from build123d import *

# Parameters (mm, degrees)
SKETCH_1_R          = 1.35
EXTRUDE_1_DEPTH     = 10
SKETCH_2_W          = 110
SKETCH_2_H          = 30
EXTRUDE_2_DEPTH     = 26
CUT_EXTRUDE_1_DEPTH = 76.432088663
EXTRUDE_3_DEPTH     = 7
SKETCH_5_R          = 1.35
CUT_EXTRUDE_2_DEPTH = 7
SKETCH_6_W          = 65
SKETCH_6_H          = 6
EXTRUDE_4_DEPTH     = 4
SKETCH_7_W          = 3.3
SKETCH_7_H          = 30
SKETCH_7_W_2        = 2.7
EXTRUDE_5_DEPTH     = 9
RIB_1_REACH         = 79.332
SKETCH_8_WALL_W     = 169.39207434
SKETCH_8_WALL_H     = 10
RIB_2_REACH         = 79.332
SKETCH_9_WALL_W     = 167.056457124
SKETCH_9_WALL_H     = 10
CUT_EXTRUDE_3_REACH = 124.7
SKETCH_10_R         = 1.75
CUT_EXTRUDE_4_REACH = 124.7
SKETCH_11_R         = 1.75
FILLET_1_R          = 2
CUT_EXTRUDE_5_DEPTH = 22
CHAMFER_1_SIZE      = 5
CHAMFER_2_SIZE      = 2
SKETCH_13_R         = 1.75
CUT_EXTRUDE_6_DEPTH = 72.973953622
CHAMFER_3_SIZE      = 5
SKETCH_14_R         = 3
CUT_EXTRUDE_7_DEPTH = 4


with BuildPart() as part:
    # 草图1 → 凸台-拉伸1 (new body)
    with BuildSketch(Plane(origin=(0, 0, 0), x_dir=(1, 0, 0), z_dir=(0, 1, 0))):
        with BuildLine():
            Line((10, 15), (55, 15))
            Line((55, 15), (55, -15))
            Line((55, -15), (10, -15))
            ThreePointArc((10, -15), (6.464466094, -16.464466094), (5, -20))
            Line((5, -20), (5, -25.5))
            ThreePointArc((5, -25.5), (3.535533906, -29.035533906), (0, -30.5))
            Line((0, -30.5), (-30, -30.5))
            ThreePointArc((-30, -30.5), (-33.535533906, -29.035533906), (-35, -25.5))
            Line((-35, -25.5), (-35, -20))
            ThreePointArc((-35, -20), (-36.464466094, -16.464466094), (-40, -15))
            Line((-40, -15), (-55, -15))
            Line((-55, -15), (-55, 15))
            Line((-55, 15), (-40, 15))
            ThreePointArc((-40, 15), (-36.464466094, 16.464466094), (-35, 20))
            Line((-35, 20), (-35, 22))
            Line((-35, 22), (5, 22))
            Line((5, 22), (5, 20))
            ThreePointArc((5, 20), (6.464466094, 16.464466094), (10, 15))
        make_face()
        with Locations(Location((-30, 14.5, 0), (0, 0, 270))):
            Circle(SKETCH_1_R, mode=Mode.SUBTRACT)
        with Locations(Location((0, 14.5, 0), (0, 0, 270))):
            Circle(SKETCH_1_R, mode=Mode.SUBTRACT)
        with Locations(Location((0, -25.5, 0), (0, 0, 270))):
            Circle(SKETCH_1_R, mode=Mode.SUBTRACT)
        with Locations(Location((-30, -25.5, 0), (0, 0, 270))):
            Circle(SKETCH_1_R, mode=Mode.SUBTRACT)
    extrude(amount=EXTRUDE_1_DEPTH)

    # 草图2 → 凸台-拉伸2 (add)
    with BuildSketch(Plane(origin=(0, 10, 0), x_dir=(1, 0, 0), z_dir=(0, 1, 0))):
        Rectangle(SKETCH_2_W, SKETCH_2_H)
    extrude(amount=EXTRUDE_2_DEPTH)

    # 草图3 → 切除-拉伸1 (cut, through all)
    with BuildSketch(Plane.XY.offset(15)):
        with BuildLine():
            Line((-42, 30), (-28, 30))
            ThreePointArc((-28, 30), (-25.878679656, 29.121320344), (-25, 27))
            Line((-25, 27), (-25, 13))
            ThreePointArc((-25, 13), (-25.878679656, 10.878679656), (-28, 10))
            Line((-28, 10), (-42, 10))
            ThreePointArc((-42, 10), (-44.121320344, 10.878679656), (-45, 13))
            Line((-45, 13), (-45, 27))
            ThreePointArc((-45, 27), (-44.121320344, 29.121320344), (-42, 30))
        make_face()
        with BuildLine():
            Line((22, 10), (46, 10))
            ThreePointArc((46, 10), (48.121320344, 10.878679656), (49, 13))
            Line((49, 13), (49, 27))
            ThreePointArc((49, 27), (48.121320344, 29.121320344), (46, 30))
            Line((46, 30), (22, 30))
            ThreePointArc((22, 30), (19.878679656, 29.121320344), (19, 27))
            Line((19, 27), (19, 13))
            ThreePointArc((19, 13), (19.878679656, 10.878679656), (22, 10))
        make_face()
    extrude(amount=-CUT_EXTRUDE_1_DEPTH, mode=Mode.SUBTRACT)

    # 草图4 → 凸台-拉伸3 (add)
    with BuildSketch(Plane(origin=(0, 36, 0), x_dir=(1, 0, 0), z_dir=(0, 1, 0))):
        with BuildLine():
            Line((-28.5, 9), (39.5, 9))
            ThreePointArc((39.5, 9), (41.267766953, 8.267766953), (42, 6.5))
            Line((42, 6.5), (42, -6.5))
            ThreePointArc((42, -6.5), (41.267766953, -8.267766953), (39.5, -9))
            Line((39.5, -9), (-28.5, -9))
            ThreePointArc((-28.5, -9), (-30.267766953, -8.267766953), (-31, -6.5))
            Line((-31, -6.5), (-31, 6.5))
            ThreePointArc((-31, 6.5), (-30.267766953, 8.267766953), (-28.5, 9))
        make_face()
    extrude(amount=EXTRUDE_3_DEPTH)

    # 草图5 → 切除-拉伸2 (cut)
    with BuildSketch(Plane(origin=(0, 36, 0), x_dir=(1, 0, 0), z_dir=(0, 1, 0))):
        with Locations(Location((43.5, 11.5, 0), (0, 0, 270))):
            Circle(SKETCH_5_R)
        with Locations(Location((43.5, -10.5, 0), (0, 0, 270))):
            Circle(SKETCH_5_R)
        with Locations(Location((-31.5, -10.5, 0), (0, 0, 270))):
            Circle(SKETCH_5_R)
        with Locations(Location((-31.5, 11.5, 0), (0, 0, 270))):
            Circle(SKETCH_5_R)
    extrude(amount=-CUT_EXTRUDE_2_DEPTH, mode=Mode.SUBTRACT)

    # 草图6 → 凸台-拉伸4 (add)
    with BuildSketch(Plane(origin=(0, 36, 0), x_dir=(1, 0, 0), z_dir=(0, 1, 0))):
        with Locations((5.5, -12)):
            Rectangle(SKETCH_6_W, SKETCH_6_H)
    extrude(amount=EXTRUDE_4_DEPTH)

    # 草图7 → 凸台-拉伸5 (add)
    with BuildSketch(Plane(origin=(0, 36, 0), x_dir=(1, 0, 0), z_dir=(0, 1, 0))):
        with Locations((-53.35, 0)):
            Rectangle(SKETCH_7_W, SKETCH_7_H)
        with Locations((53.65, 0)):
            Rectangle(SKETCH_7_W_2, SKETCH_7_H)
    extrude(amount=EXTRUDE_5_DEPTH)

    # 草图8 wall → 筋1 (add, up to next)
    with BuildSketch(Plane(origin=(-47.2, 40.5, 0), x_dir=(0.707106781187, -0.707106781187, 0), z_dir=(0.707106781187, 0.707106781187, 0)), mode=Mode.PRIVATE) as rib_1_sk1:
        Rectangle(SKETCH_8_WALL_W, SKETCH_8_WALL_H)
    rib_1_tool1 = extrude(rib_1_sk1.sketch, amount=-RIB_1_REACH, mode=Mode.PRIVATE) - part.part
    add(rib_1_tool1.solids().sort_by_distance((-47.2, 40.5, 0))[0])

    # 草图9 wall → 筋2 (add, up to next)
    with BuildSketch(Plane(origin=(49.701923788, 40.5, 0), x_dir=(-0.500000000021, -0.866025403772, 0), z_dir=(0.866025403772, -0.500000000021, 0)), mode=Mode.PRIVATE) as rib_2_sk1:
        Rectangle(SKETCH_9_WALL_W, SKETCH_9_WALL_H)
    rib_2_tool1 = extrude(rib_2_sk1.sketch, amount=RIB_2_REACH, mode=Mode.PRIVATE) - part.part
    add(rib_2_tool1.solids().sort_by_distance((49.701923788, 40.5, 0))[0])

    # 草图10 → 切除-拉伸3 (cut, up to next)
    with BuildSketch(Plane(origin=(55, 0, 0), x_dir=(0, 0, -1), z_dir=(1, 0, 0)), mode=Mode.PRIVATE) as cut_extrude_3_sk1:
        with Locations((-10.5, 41.5)):
            Circle(SKETCH_10_R)
    cut_extrude_3_tool1 = extrude(cut_extrude_3_sk1.sketch, amount=-CUT_EXTRUDE_3_REACH, mode=Mode.PRIVATE) & part.part
    # 草图10 → 切除-拉伸3 (cut, up to next)
    with BuildSketch(Plane(origin=(55, 0, 0), x_dir=(0, 0, -1), z_dir=(1, 0, 0)), mode=Mode.PRIVATE) as cut_extrude_3_sk2:
        with Locations((7.5, 41.5)):
            Circle(SKETCH_10_R)
    cut_extrude_3_tool2 = extrude(cut_extrude_3_sk2.sketch, amount=-CUT_EXTRUDE_3_REACH, mode=Mode.PRIVATE) & part.part
    add(cut_extrude_3_tool1.solids().sort_by_distance((55, 41.5, 10.5))[0], mode=Mode.SUBTRACT)
    add(cut_extrude_3_tool2.solids().sort_by_distance((55, 41.5, -7.5))[0], mode=Mode.SUBTRACT)

    # 草图11 → 切除-拉伸4 (cut, up to next)
    with BuildSketch(Plane.ZY.offset(55), mode=Mode.PRIVATE) as cut_extrude_4_sk1:
        with Locations(Location((10.5, 41.5, 0), (0, 0, 180))):
            Circle(SKETCH_11_R)
    cut_extrude_4_tool1 = extrude(cut_extrude_4_sk1.sketch, amount=-CUT_EXTRUDE_4_REACH, mode=Mode.PRIVATE) & part.part
    # 草图11 → 切除-拉伸4 (cut, up to next)
    with BuildSketch(Plane.ZY.offset(55), mode=Mode.PRIVATE) as cut_extrude_4_sk2:
        with Locations((-11.5, 41.5)):
            Circle(SKETCH_11_R)
    cut_extrude_4_tool2 = extrude(cut_extrude_4_sk2.sketch, amount=-CUT_EXTRUDE_4_REACH, mode=Mode.PRIVATE) & part.part
    add(cut_extrude_4_tool1.solids().sort_by_distance((-55, 41.5, 10.5))[0], mode=Mode.SUBTRACT)
    add(cut_extrude_4_tool2.solids().sort_by_distance((-55, 41.5, -11.5))[0], mode=Mode.SUBTRACT)

    # 圆角1
    fillet_1_edges = [part.edges().sort_by_distance(p)[0] for p in [
        (-27, 36, 12),
        (38, 36, 12),
    ]]
    fillet(fillet_1_edges, radius=FILLET_1_R)

    # 草图12 → 切除-拉伸5 (cut)
    with BuildSketch(Plane(origin=(0, 43, 0), x_dir=(1, 0, 0), z_dir=(0, 1, 0))):
        Polygon((-22, -15), (-22, 15), (16, 15), (16, 8), (1, 2), (1, -15), align=None)
    extrude(amount=-CUT_EXTRUDE_5_DEPTH, mode=Mode.SUBTRACT)

    # 倒角1
    chamfer_1_edges = [part.edges().sort_by_distance(p)[0] for p in [
        (-55, 0, 0),
    ]]
    chamfer(chamfer_1_edges, length=CHAMFER_1_SIZE)

    # 倒角2
    chamfer_2_edges = [part.edges().sort_by_distance(p)[0] for p in [
        (-53.35, 45, 15),
        (-53.35, 45, -15),
        (53.65, 45, -15),
        (53.65, 45, 15),
    ]]
    chamfer(chamfer_2_edges, length=CHAMFER_2_SIZE)

    # 草图13 → 切除-拉伸6 (cut, through all)
    with BuildSketch(Plane(origin=(0, 10, 0), x_dir=(1, 0, 0), z_dir=(0, 1, 0))):
        with Locations(Location((43.5, 11.5, 0), (0, 0, 270))):
            Circle(SKETCH_13_R)
        with Locations(Location((43.5, -10.5, 0), (0, 0, 270))):
            Circle(SKETCH_13_R)
        with Locations(Location((-31.5, 11.5, 0), (0, 0, 270))):
            Circle(SKETCH_13_R)
        with Locations(Location((-31.5, -10.5, 0), (0, 0, 270))):
            Circle(SKETCH_13_R)
    extrude(amount=-CUT_EXTRUDE_6_DEPTH, mode=Mode.SUBTRACT)

    # 倒角3
    chamfer_3_edges = [part.edges().sort_by_distance(p)[0] for p in [
        (55, 0, 0),
    ]]
    chamfer(chamfer_3_edges, length=CHAMFER_3_SIZE)

    # 草图14 → 切除-拉伸7 (cut)
    with BuildSketch(Plane.XZ):
        with Locations((20, -14.5)):
            Circle(SKETCH_14_R)
    extrude(amount=-CUT_EXTRUDE_7_DEPTH, mode=Mode.SUBTRACT)


solid = part.part
Could you check a few things on this model? Use its own coordinates, in mm. A direction names the side the tool comes from. Coordinates: 2 decimals unless noted, no trailing zeros. Loops run counter-clockwise (first coordinate to the right, second up) from the corner with the lowest first, then second, coordinate; pieces in that order, holes last. Notation, with made-up numbers: (1.25, -11.5) -> (46.25, -11.5) arc R4 ccw to (46.25, -6.5) -> close; hole circle Ø8 at (19.5, -15). An arc over 180 degrees is marked (long way). Answer in a Markdown table with one row per item.
(1) Imagine slicing it at A-A (x = 36.5). List the corners of the cut face in (y, z) for me, plus the area to 3 significant figures.
Results found:
| item | result |
|---|---|
| outline | (0, -15) -> (10, -15) -> (10, 15) -> (0, 15) -> close; (30, -15) -> (36, -15) -> (36, -9) -> (43, -9) -> (43, 9) -> (40, 9) -> (40, 15) -> (30, 15) -> close |
| area | 630 mm^2 |
(2) If I drill on probe 1 along X at (y, z) = (15, 11); probe 2 along X at (y, z) = (32.65, 10.5); probe 3 along X at (y, z) = (2, 10.5), over which ranges is the centre line in solid material (lowest first)?
Results found:
| item | result |
|---|---|
| probe 1 | x = -55 to -45, -25 to 19, 49 to 55 |
| probe 2 | x = -55 to -32.85, -30.15 to -22, 1 to 42.15, 44.85 to 55 |
| probe 3 | x = -52 to -33.25, -29.75 to 41.75, 45.25 to 52 |
(3) Imagine slicing it at C-C (y = 7). Give the number of separate pieces and of enclosed holes in the cut face, plus the area to 3 significant figures.
Results found:
| item | result |
|---|---|
| separate pieces | 1 |
| enclosed holes | 8 |
| area | 4,150 mm^2 |
(4) Thinking about a two-plate mould opening in Y: for faces 5 (the face through (20, 4, -14)), 6 (the face through (-25, 39, -9)), 7 (the face through (-53.37, 39.79, -11.88)), which applies, released by +Y, released by -Y, zero draft, split by the parting line, or undercut?
Results found:
| item | result |
|---|---|
| face 5 | released by -Y |
| face 6 | zero draft |
| face 7 | undercut |
(5) Will these pins go through, and if not, where does the flat tip stop? pin 1 Ø3.5 at (x, z) = (0, 25.5) entering from +Y; pin 2 Ø2 at (x, z) = (-7.5, -7) entering from +Y; pin 3 Ø2 at (x, z) = (43.5, -11.5) entering from +Y; pin 4 Ø12 at (y, z) = (13.5, 20.5) entering from +X.
Results found:
| item | result |
|---|---|
| pin 1 | stops at y = 10 |
| pin 2 | stops at y = 21 |
| pin 3 | passes through |
| pin 4 | stops at x = 55 |
(6) Imagine slicing it at B-B (y = 16). List the corners of the cut face in (x, z) for me.
Results found:
| item | result |
|---|---|
| outline | (-55, -15) -> (-45, -15) -> (-45, 15) -> (-55, 15) -> close; (-25, -15) -> (19, -15) -> (19, 15) -> (-25, 15) -> close; (49, -15) -> (55, -15) -> (55, 15) -> (49, 15) -> close |
(7) For faces 1 (the face through (0.06, 4.93, -15.85)), 2 (the face through (-44.14, 29.1, 0.21)), 3 (the face through (52.3, 39, 10)), 4 (the face through (-40, 36, 0)), which set-ups out of +Z, -Z, +X, -X, +Y, -Y let a thin tool reach every point of the face, with its end or its side?
Results found:
| item | result |
|---|---|
| face 1 | -Y |
| face 2 | +Z, -Z |
| face 3 | +Z, +Y |
| face 4 | +Y |
